Autodesk Inventor part; units mm, degrees
ref_plane "YZ Plane" through (0, 0, 0) normal (1, 0, 0) x (0, 1, 0)
ref_plane "XZ Plane" through (0, 0, 0) normal (0, 1, 0) x (-1, 0, 0)
ref_plane "XY Plane" through (0, 0, 0) normal (0, 0, 1) x (1, 0, 0)
sketch "スケッチ1" plane through (0, 0, 0) normal (0, 0, 1) x (1, 0, 0)
  circle A0 centre (0, 0) radius 25.25
  circle A1 centre (0, 0) radius 20.25
  dimension "d0" = 5
  dimension "d1" = 40.5
extrude "押し出し1" add sketch "スケッチ1" along normal blind 8
sketch "スケッチ2" plane through (0, 0, 0) normal (0, 0, 1) x (1, 0, 0)
  circle A0 centre (0, 0) radius 25.25
  arc A1 (8.2256, -22.5996) -> (8.2256, 22.5996) centre (0, 0) ccw
  line L0 (0, -35.35) -> (0, 35.35)
  line L1 (8.2256, 22.5996) -> (8.636, 23.7272)
  line L2 (8.2256, -22.5996) -> (8.636, -23.7272)
  line L3 (-35.35, 0) -> (35.35, 0)
  point P0 (24.05, 0)
  dimension "d4" = 1.2
  dimension "d5" = 140
extrude "押し出し2" cut sketch "スケッチ2" along normal blind 5 contours L3 A1 L1 A0 | A0 L2 A1 L3
mirror "ミラー1" about plane through (0, 0, 0) normal (1, 0, 0) of "押し出し2"
sketch "スケッチ4" plane through (0, 0, 8) normal (0, 0, 1) x (1, 0, 0)
  circle A0 centre (0, 0) radius 25.25
  line L0 (21.7123, -12.5356) -> (0, 0)
  line L1 (-35.8782, 0) -> (38.5193, 0)
  arc A1 (23.8972, -19.3516) -> (28.7076, -11.0198) centre (0, 0) ccw
  arc A2 (17.6801, -14.317) -> (21.239, -8.1529) centre (0, 0) ccw
  line L2 (23.8972, -19.3516) -> (17.6801, -14.317)
  line L3 (21.239, -8.1529) -> (28.7076, -11.0198)
  circle A3 centre (0, 0) radius 20.25
  point P0 (26.6303, -15.375)
  point P1 (19.7021, -11.375)
  dimension "d18" = 30
  dimension "d46" = 2.5
  dimension "d47" = 8
  dimension "d48" = 18
extrude "押し出し7" add sketch "スケッチ4" along normal blind 2.5 and the other way blind 1 contours L3 A1 L2 A0 | A0 L2 A2 L3
chamfer "面取り4" distance 2.5 angle 45 1 edges at (19.7021, -11.375, 8)
sketch "スケッチ7" plane through (0, 0, 8) normal (0, 0, 1) x (1, 0, 0)
  arc A0 (23.7272, -8.636) -> (19.3426, -16.2304) centre (0, 0) ccw
  arc A1 (21.472, -7.8152) -> (17.5041, -14.6877) centre (0, 0) ccw
  arc A2 (18.905, -7.257) -> (15.7372, -12.7437) centre (0, 0) ccw
  line L0 (21.472, -7.8152) -> (23.7272, -8.636)
  arc A3 (23.5729, -9.0488) -> (19.6229, -15.8903) centre (0, 0) ccw
  line L1 (17.5041, -14.6877) -> (19.3426, -16.2304)
  line L2 (17.6801, -14.317) -> (23.8972, -19.3516)
  line L3 (28.7076, -11.0198) -> (21.239, -8.1529)
  dimension "d57" = 1
  dimension "d59" = 2.4
  dimension "d65" = 1
extrude "押し出し8" cut sketch "スケッチ7" against normal blind 3
chamfer "面取り5" distance 1.5 angle 45 3 edges at (26.6303, -15.375, 10.5) (24.9733, -9.5863, 10.5) (20.7887, -16.8343, 10.5)
properties part number "ring"
Geometry: final body of the model. Coordinates: model frame, mm. A direction names the side the tool comes from. Give positions to 0.01 mm unless a question says otherwise; leave off trailing zeros. Write each loop counter-clockwise with the first axis right and the second up, starting at its lowest first coordinate (ties: lowest second). Pieces come first, ordered by that corner, then holes.
(1) Mould query, pull axis Y, two halves, no side actions, for faces 5 (the flat face through (23, -13, 10.5)), 6 (the flat face through (20.781, -16.828, 8.208)), 7 (the cylindrical face through (11, -17, 4)). Classes: released by +Y, released by -Y, zero draft, split by the parting line, or undercut.
(2) Access query for faces 1 (the flat face through (-18, -15, 5)), 2 (the flat face through (8.43, -23.16, 2.46)), 3 (the flat face through (-8.434, -23.171, 2.465)), 4 (the flat face through (21.3, -12.2, 5)). Directions: +Z, -Z, +X, -X, +Y, -Y. A direction counts if a zero-diameter tool reaches every point of the face in a straight line with its end or side. Return the directions, or none.
(3) Cut plane A-A, the plane x = 0. Return loops of the section in (y, z), then the cut area to 3 significant figures.
(4) Ray query, line 1 (X direction, y = 0, z = 4.25); line 2 (Y direction, x = 0, z = 4); line 3 (Z direction, x = -9, y = 22). Return the intervals inside material, ascending.
(5) Cut plane C-C, the plane z = 1.25. Return loops of the section in (x, y).
(6) Cut plane B-B, the plane y = 0. Return loops of the section in (x, z), then the cut area to 3 significant figures.
(7) First-contact query: P1, Ø2.5, axis at x = 22.5, y = -15, coming from the -Z side; P2, Ø6, axis at y = 5, z = 8.5, coming from the -X side; P3, Ø5, axis at y = -16.5, z = 6.5, coming from the -X side; P4, Ø13.5, axis at x = -4.5, y = -7.5, coming from the +Z side. Flat tips, straight axial feed; report the tip coordinate or a pass-through.
Values follow:
1. face 5: zero draft
1. face 6: released by -Y
1. face 7: undercut
2. face 1: +Z
2. face 2: +Z, -Z, +X
2. face 3: +Z, -Z, -X
2. face 4: -Z, +X, -Y
3. outline: (-25.25, 0) - (-20.25, 0) - (-20.25, 8) - (-22.85, 8) - (-22.85, 5) - (-25.25, 5) - close; (20.25, 0) - (25.25, 0) - (25.25, 5) - (22.85, 5) - (22.85, 8) - (20.25, 8) - close
3. area: 65.6 mm2
4. line 1: x = -24.05 to -20.25, 20.25 to 24.05
4. line 2: y = -25.25 to -20.25, 20.25 to 25.25
4. line 3: z = 0 to 5
5. outline: (-8.64, -23.73) arc R25.25 ccw to (8.64, -23.73) - (8.23, -22.6) arc R24.05 ccw to (8.23, 22.6) - (8.64, 23.73) arc R25.25 ccw to (-8.64, 23.73) - (-8.23, 22.6) arc R24.05 ccw to (-8.23, -22.6) - close; hole circle Ø40.5 at (0, 0)
6. outline: (-24.05, 0) - (-20.25, 0) - (-20.25, 8) - (-22.85, 8) - (-22.85, 5) - (-24.05, 5) - close; (20.25, 0) - (24.05, 0) - (24.05, 5) - (22.85, 5) - (22.85, 8) - (20.25, 8) - close
6. area: 53.6 mm2
7. P1: stops at z = 7
7. P2: stops at x = -22.76
7. P3: stops at x = -19.19
7. P4: passes through
